```python
from build123d import *

# Parameters (mm, degrees)
F0_R     = 15
F1_DEPTH = 25


with BuildPart() as f1:
    # F0 (on Right) → F1 (new body)
    with BuildSketch(Plane.YZ):
        with BuildLine():
            Line((-40, 102.469508), (-40, -102.469508))
            ThreePointArc((-40, -102.469508), (0, -110), (40, -102.469508))
            Line((40, -102.469508), (40, 102.469508))
            ThreePointArc((40, 102.469508), (0, 110), (-40, 102.469508))
        make_face()
        with Locations((0, -75)):
            Circle(F0_R, mode=Mode.SUBTRACT)
        with Locations((0, 75)):
            Circle(F0_R, mode=Mode.SUBTRACT)
    extrude(amount=F1_DEPTH)


solid = f1.part
```
Work out the finished part from the listing and answer in its coordinate system (mm). Round coordinates to 2 decimals unless told otherwise and drop trailing zeros. Loops run counter-clockwise (first coordinate to the right, second up) from the corner with the lowest first, then second, coordinate; pieces in that order, holes last. Notation, with made-up numbers: M 63,55.5 L 110,55.5 A14 cw 110,79.5 Z; hole C -28.5,59.5 d1. An arc over 180 degrees is marked long. Use CSV: the item, a comma, the result in double quotes.
Q1. Section D-D, the plane z = 64 is taken. Determine the outline of the cut face in (x, y), then the cut area to 3 significant figures.
Determined:
outline,"M 0,-40 L 25,-40 L 25,-10.2 L 0,-10.2 Z; M 0,10.2 L 25,10.2 L 25,40 L 0,40 Z"
area,"1,490 mm2"
Q2. Each of these flat-tipped pins is pushed along its axis until it touches: pin 1 (1.5 mm diameter, centred on x = 2.5, y = 4, fed in from -Z); pin 2 (2 mm diameter, centred on x = 19, y = -2.5, fed in from -Z); pin 3 (1 mm diameter, centred on x = 4.5, y = -9, fed in from +Z). Where does it stop, or does it pass through?
Determined:
pin 1,"z = -109.95"
pin 2,"z = -109.99"
pin 3,"z = 109.67"
Q3. Section C-C, the plane x = 7.5 is taken. Determine the outline of the cut face in (y, z).
Determined:
outline,"M -40,-102.47 A110 ccw 40,-102.47 L 40,102.47 A110 ccw -40,102.47 Z; hole C 0,-75 d30; hole C 0,75 d30"
Q4. Consider L1, parallel to Z at x = 14.5, y = 0; L2, parallel to Z at x = 21.5, y = 5; L3, parallel to Y at x = 9.5, z = -82. Determine where each line is inside the solid, lowest interval first.
Determined:
L1,"-110 to -90, -60 to 60, 90 to 110"
L2,"-109.89 to -89.14, -60.86 to 60.86, 89.14 to 109.89"
L3,"-40 to -13.27, 13.27 to 40"
Q5. Section B-B, the plane z = -75 is taken. Determine the outline of the cut face in (x, y).
Determined:
outline,"M 0,-40 L 25,-40 L 25,-15 L 0,-15 Z; M 0,15 L 25,15 L 25,40 L 0,40 Z"
Q6. The mould has two halves that part along Z. Classify faces 1 (the cylindrical face through (12.325, -3.252, 60.357)), 2 (the flat face through (25, -1, 2)), 3 (the cylindrical face through (12.325, -3.252, -89.643)), 4 (the cylindrical face through (12.3, -0.6, -110)): pulls with the +Z half, pulls with the -Z half, needs draft (parallel to the pull), parting line crosses it, or undercut.
Determined:
face 1,"undercut"
face 2,"needs draft"
face 3,"undercut"
face 4,"pulls with the -Z half"
Q7. Section A-A, the plane y = 0 is taken. Determine the outline of the cut face in (x, z), then the cut area to 3 significant figures.
Determined:
outline,"M 0,-110 L 25,-110 L 25,-90 L 0,-90 Z; M 0,-60 L 25,-60 L 25,60 L 0,60 Z; M 0,90 L 25,90 L 25,110 L 0,110 Z"
area,"4,000 mm2"
